Source: CAD feature listing. Evaluate the final solid. Frame: model axes, mm. A direction names the side the tool comes from. Give positions to 0.01 mm unless a question says otherwise; leave off trailing zeros. Order: outer loops, then holes, each group sorted by start corner. A loop starts at its lowest first (then second) coordinate and runs counter-clockwise, first axis right, second up.
from build123d import *

# Parameters (mm, degrees)
F0_R     = 9.75
F2_DEPTH = 18
F1_R     = 11.25
F1_R_2   = 9.75
F3_DEPTH = 18
F4_DEPTH = 10
F5_DEPTH = 3.2
F6_R     = 3.5
F7_DEPTH = 14.801
F9_DEPTH = 0.5


with BuildPart() as f2:
    # F0 (on Right) → F2 (new body)
    with BuildSketch(Plane.YZ):
        Circle(F0_R)
    extrude(amount=F2_DEPTH)

    # F4 (cut): a face of the model
    f4_faces = [f2.faces().sort_by_distance(p)[0] for p in [
        (0, 0, 0),
    ]]
    extrude(f4_faces, amount=-F4_DEPTH, mode=Mode.SUBTRACT)

    # F5 (cut): a face of the model
    f5_faces = [f2.faces().sort_by_distance(p)[0] for p in [
        (18, 0, 0),
    ]]
    extrude(f5_faces, amount=-F5_DEPTH, mode=Mode.SUBTRACT)

    # F6 (on face) → F7 (cut, through all)
    with BuildSketch(Plane.YZ.offset(14.8)):
        Circle(F6_R)
    extrude(amount=-F7_DEPTH, mode=Mode.SUBTRACT)



with BuildPart() as f3:
    # F1 (on face) → F3 (new body)
    with BuildSketch(Plane.YZ):
        Circle(F1_R)
        Circle(F1_R_2, mode=Mode.SUBTRACT)
    extrude(amount=F3_DEPTH)


with BuildPart() as f2_1:
    add(f2.part)

    add(f3.part)  # F9 merges F3
    # F8 (on face) → F9 (join)
    with BuildSketch(Plane.YZ.offset(14.8)):
        with BuildLine():
            ThreePointArc((-4.19606186, 3.8323562574), (-4.0183261202, 4.0183261202), (-3.8323562574, 4.19606186))
            Line((-3.8323562574, 4.19606186), (-6.1766101499, 7.5440033839))
            ThreePointArc((-6.1766101499, 7.5440033839), (-6.8942911166, 6.8942911166), (-7.5440033839, 6.1766101499))
            Line((-7.5440033839, 6.1766101499), (-4.19606186, 3.8323562574))
        make_face()
        with BuildLine():
            ThreePointArc((-2.410076423, 5.1463988625), (-2.1747024254, 5.2501960894), (-1.9348721525, 5.3432349162))
            Line((-1.9348721525, 5.3432349162), (-2.8194785891, 9.3334366921))
            ThreePointArc((-2.8194785891, 9.3334366921), (-3.7311634656, 9.007825442), (-4.606063947, 8.5934088065))
            Line((-4.606063947, 8.5934088065), (-2.410076423, 5.1463988625))
        make_face()
        with BuildLine():
            ThreePointArc((-0.2571786979, 5.676948893), (0, 5.6827712972), (0.2571786979, 5.676948893))
            Line((0.2571786979, 5.676948893), (0.9668930283, 9.7019388718))
            ThreePointArc((0.9668930283, 9.7019388718), (0, 9.75), (-0.9668930283, 9.7019388718))
            Line((-0.9668930283, 9.7019388718), (-0.2571786979, 5.676948893))
        make_face()
        with BuildLine():
            Line((2.8194785891, 9.3334366921), (1.9348721525, 5.3432349162))
            ThreePointArc((1.9348721525, 5.3432349162), (2.1747024254, 5.2501960894), (2.410076423, 5.1463988625))
            Line((2.410076423, 5.1463988625), (4.606063947, 8.5934088065))
            ThreePointArc((4.606063947, 8.5934088065), (3.7311634656, 9.007825442), (2.8194785891, 9.3334366921))
        make_face()
        with BuildLine():
            Line((6.1766101499, 7.5440033839), (3.8323562574, 4.19606186))
            ThreePointArc((3.8323562574, 4.19606186), (4.0183261202, 4.0183261202), (4.19606186, 3.8323562574))
            Line((4.19606186, 3.8323562574), (7.5440033839, 6.1766101499))
            ThreePointArc((7.5440033839, 6.1766101499), (6.8942911166, 6.8942911166), (6.1766101499, 7.5440033839))
        make_face()
        with BuildLine():
            Line((8.5934088065, 4.606063947), (5.1463988625, 2.410076423))
            ThreePointArc((5.1463988625, 2.410076423), (5.2501960894, 2.1747024254), (5.3432349162, 1.9348721525))
            Line((5.3432349162, 1.9348721525), (9.3334366921, 2.8194785891))
            ThreePointArc((9.3334366921, 2.8194785891), (9.007825442, 3.7311634656), (8.5934088065, 4.606063947))
        make_face()
        with BuildLine():
            Line((9.7019388718, 0.9668930283), (5.676948893, 0.2571786979))
            ThreePointArc((5.676948893, 0.2571786979), (5.6813155097, 0.1286222989), (5.6827712972, 0))
            ThreePointArc((5.6827712972, 0), (5.6813155097, -0.1286222989), (5.676948893, -0.2571786979))
            Line((5.676948893, -0.2571786979), (9.7019388718, -0.9668930283))
            ThreePointArc((9.7019388718, -0.9668930283), (9.7379773054, -0.4840433865), (9.75, 0))
            ThreePointArc((9.75, 0), (9.7379773054, 0.4840433865), (9.7019388718, 0.9668930283))
        make_face()
        with BuildLine():
            Line((9.3334366921, -2.8194785891), (5.3432349162, -1.9348721525))
            ThreePointArc((5.3432349162, -1.9348721525), (5.2501960894, -2.1747024254), (5.1463988625, -2.410076423))
            Line((5.1463988625, -2.410076423), (8.5934088065, -4.606063947))
            ThreePointArc((8.5934088065, -4.606063947), (9.007825442, -3.7311634656), (9.3334366921, -2.8194785891))
        make_face()
        with BuildLine():
            Line((7.5440033839, -6.1766101499), (4.19606186, -3.8323562574))
            ThreePointArc((4.19606186, -3.8323562574), (4.0183261202, -4.0183261202), (3.8323562574, -4.19606186))
            Line((3.8323562574, -4.19606186), (6.1766101499, -7.5440033839))
            ThreePointArc((6.1766101499, -7.5440033839), (6.8942911166, -6.8942911166), (7.5440033839, -6.1766101499))
        make_face()
        with BuildLine():
            Line((4.606063947, -8.5934088065), (2.410076423, -5.1463988625))
            ThreePointArc((2.410076423, -5.1463988625), (2.1747024254, -5.2501960894), (1.9348721525, -5.3432349162))
            Line((1.9348721525, -5.3432349162), (2.8194785891, -9.3334366921))
            ThreePointArc((2.8194785891, -9.3334366921), (3.7311634656, -9.007825442), (4.606063947, -8.5934088065))
        make_face()
        with BuildLine():
            ThreePointArc((0.2571786979, -5.676948893), (0, -5.6827712972), (-0.2571786979, -5.676948893))
            Line((-0.2571786979, -5.676948893), (-0.9668930283, -9.7019388718))
            ThreePointArc((-0.9668930283, -9.7019388718), (0, -9.75), (0.9668930283, -9.7019388718))
            Line((0.9668930283, -9.7019388718), (0.2571786979, -5.676948893))
        make_face()
        with BuildLine():
            ThreePointArc((-1.9348721525, -5.3432349162), (-2.1747024254, -5.2501960894), (-2.410076423, -5.1463988625))
            Line((-2.410076423, -5.1463988625), (-4.606063947, -8.5934088065))
            ThreePointArc((-4.606063947, -8.5934088065), (-3.7311634656, -9.007825442), (-2.8194785891, -9.3334366921))
            Line((-2.8194785891, -9.3334366921), (-1.9348721525, -5.3432349162))
        make_face()
        with BuildLine():
            ThreePointArc((-3.8323562574, -4.19606186), (-4.0183261202, -4.0183261202), (-4.19606186, -3.8323562574))
            Line((-4.19606186, -3.8323562574), (-7.5440033839, -6.1766101499))
            ThreePointArc((-7.5440033839, -6.1766101499), (-6.8942911166, -6.8942911166), (-6.1766101499, -7.5440033839))
            Line((-6.1766101499, -7.5440033839), (-3.8323562574, -4.19606186))
        make_face()
        with BuildLine():
            ThreePointArc((-5.1463988625, -2.410076423), (-5.2501960894, -2.1747024254), (-5.3432349162, -1.9348721525))
            Line((-5.3432349162, -1.9348721525), (-9.3334366921, -2.8194785891))
            ThreePointArc((-9.3334366921, -2.8194785891), (-9.007825442, -3.7311634656), (-8.5934088065, -4.606063947))
            Line((-8.5934088065, -4.606063947), (-5.1463988625, -2.410076423))
        make_face()
        with BuildLine():
            ThreePointArc((-5.676948893, -0.2571786979), (-5.6827712972, 0), (-5.676948893, 0.2571786979))
            Line((-5.676948893, 0.2571786979), (-9.7019388718, 0.9668930283))
            ThreePointArc((-9.7019388718, 0.9668930283), (-9.75, 0), (-9.7019388718, -0.9668930283))
            Line((-9.7019388718, -0.9668930283), (-5.676948893, -0.2571786979))
        make_face()
        with BuildLine():
            ThreePointArc((-5.3432349162, 1.9348721525), (-5.2501960894, 2.1747024254), (-5.1463988625, 2.410076423))
            Line((-5.1463988625, 2.410076423), (-8.5934088065, 4.606063947))
            ThreePointArc((-8.5934088065, 4.606063947), (-9.007825442, 3.7311634656), (-9.3334366921, 2.8194785891))
            Line((-9.3334366921, 2.8194785891), (-5.3432349162, 1.9348721525))
        make_face()
    extrude(amount=F9_DEPTH)


solid = f2_1.part
1) Section query A-A on x = 7.75. Output: boundary loops of the cut face in (y, z), and give its area (3 significant figures).
Checks:
outline: circle Ø22.5 at (0, 0); hole circle Ø19.5 at (0, 0)
area: 99.0 mm2
2) First-contact query: pin 1 Ø5 at (x, z) = (8, 5.5) entering from -Y; pin 2 Ø8 at (x, y) = (6.5, -5) entering from +Z; pin 3 Ø1 at (y, z) = (8, 0) entering from +X. Flat tips, straight axial feed; report the tip coordinate or a pass-through.
Checks:
pin 1: stops at y = -10.84
pin 2: stops at z = 11.21
pin 3: stops at x = 15.3
3) Section query D-D on x = 13.75. Output: boundary loops of the cut face in (y, z).
Checks:
outline: circle Ø22.5 at (0, 0); hole circle Ø7 at (0, 0)
4) Reachability of faces 3 (the face through (12.434, 3.233, -1.341)), 4 (the face through (15.046, -3.493, -6.846)) from +Z, -Z, +X, -X, +Y, -Y: full face, straight path, thin tool, end or side. Return the list, or none.
Checks:
face 3: +X, -X
face 4: +X
5) Ray query, L1, parallel to Z at x = 3.25, y = 0; L2, parallel to X at y = -8.5, z = -2.5; L3, parallel to Y at x = 5.25, z = -5.75. Return the intervals inside material, ascending.
Checks:
L1: z = -11.25 to -9.75, 9.75 to 11.25
L2: x = 10 to 14.8
L3: y = -9.67 to -7.87, 7.87 to 9.67
6) Section query B-B on z = 6.5. Output: boundary loops of the cut face in (x, y).
Checks:
outline: (0, -9.18) - (18, -9.18) - (18, -7.27) - (15.3, -7.27) - (15.3, -5.45) - (14.8, -5.45) - (14.8, -3.27) - (15.3, -3.27) - (15.3, -2.19) - (14.8, -2.19) - (14.8, -0.4) - (15.3, -0.4) - (15.3, 0.4) - (14.8, 0.4) - (14.8, 2.19) - (15.3, 2.19) - (15.3, 3.27) - (14.8, 3.27) - (14.8, 5.45) - (15.3, 5.45) - (15.3, 7.27) - (18, 7.27) - (18, 9.18) - (0, 9.18) - (0, 7.27) - (10, 7.27) - (10, -7.27) - (0, -7.27) - close
7) Pull-direction query (Z, two-part tool) for faces 1 (the face through (15.05, 5.89, -5.02)), 2 (the face through (18, 0, 10)); classes: +Z half, -Z half, draft (parallel to the pull), parting line (faces both ways), or undercut.
Checks:
face 1: undercut
face 2: draft
